```python
from build123d import *

# Parameters (mm, degrees)
SKETCH1_R           = 11
SKETCH1_R_2         = 9.652
BOSS_EXTRUDE1_DEPTH = 15
BOSS_EXTRUDE2_START = 1.5
SKETCH2_R           = 11
BOSS_EXTRUDE2_DEPTH = 1.5
SKETCH4_W           = 5
SKETCH4_H           = 12
BOSS_EXTRUDE4_DEPTH = 35
SKETCH5_R           = 4
CUT_EXTRUDE1_DEPTH  = 5
CUT_EXTRUDE2_DEPTH  = 41.441315508
FILLET1_R           = 4


with BuildPart() as part:
    # Sketch1 → Boss-Extrude1 (new body)
    with BuildSketch(Plane(origin=(0, 0, 0), x_dir=(1, 0, 0), z_dir=(0, 1, 0))):
        with Locations(Location((0, 0, 0), (0, 0, 270))):
            Circle(SKETCH1_R)
        with Locations(Location((0, 0, 0), (0, 0, 270))):
            Circle(SKETCH1_R_2, mode=Mode.SUBTRACT)
    extrude(amount=BOSS_EXTRUDE1_DEPTH)

    # Sketch2 → Boss-Extrude2 (add)
    with BuildSketch(Plane.XZ.offset(BOSS_EXTRUDE2_START)):
        with Locations(Location((0, 0, 0), (0, 0, 270))):
            Circle(SKETCH2_R)
    extrude(amount=-BOSS_EXTRUDE2_DEPTH)

    # Sketch4 → Boss-Extrude4 (add)
    with BuildSketch(Plane.XZ.offset(1.5)):
        Rectangle(SKETCH4_W, SKETCH4_H)
    extrude(amount=BOSS_EXTRUDE4_DEPTH)

    # Sketch5 → Cut-Extrude1 (cut)
    with BuildSketch(Plane.ZY.offset(2.5)):
        with Locations((0, -30.5)):
            Circle(SKETCH5_R)
    extrude(amount=-CUT_EXTRUDE1_DEPTH, mode=Mode.SUBTRACT)

    # Sketch6 → Cut-Extrude2 (cut, through all)
    with BuildSketch(Plane.ZY.offset(2.5)):
        with BuildLine():
            Line((-6, -30.5), (-6, -36.5))
            ThreePointArc((-6, -36.5), (0, -38.985281374), (6, -36.5))
            Line((6, -36.5), (6, -30.5))
            ThreePointArc((6, -30.5), (0, -36.5), (-6, -30.5))
        make_face()
    extrude(amount=-CUT_EXTRUDE2_DEPTH, mode=Mode.SUBTRACT)

    # Fillet1
    # the kernel refuses this fillet: 4 mm, written as the material it adds along each edge
    with BuildSketch(Plane(origin=(2.5, -1.5, -6), x_dir=(1, 0, 0), z_dir=(0, 0, 1)), Plane(origin=(-2.5, -1.5, 6), x_dir=(-1, 0, 0), z_dir=(0, 0, -1))) as fillet1_piece_1:
        with BuildLine():
            CenterArc((FILLET1_R, -FILLET1_R), FILLET1_R, 90, 90)
            Line((0, -FILLET1_R), (0, 0))
            Line((0, 0), (FILLET1_R, 0))
        make_face()
    extrude(amount=12)
    with BuildSketch(Plane(origin=(2.5, -1.5, 6), x_dir=(0, 0, 1), z_dir=(-1, 0, 0)), Plane(origin=(-2.5, -1.5, -6), x_dir=(0, 0, -1), z_dir=(1, 0, 0))) as fillet1_piece_2:
        with BuildLine():
            CenterArc((FILLET1_R, -FILLET1_R), FILLET1_R, 90, 90)
            Line((0, -FILLET1_R), (0, 0))
            Line((0, 0), (FILLET1_R, 0))
        make_face()
    extrude(amount=5)
    with BuildSketch(Plane(origin=(-2.5, -1.5, -6), x_dir=(0, 0, -1), z_dir=(1, 0, 0))) as fillet1_piece_3a_section:
        with BuildLine():
            CenterArc((FILLET1_R, -FILLET1_R), FILLET1_R, 90, 90)
            Line((0, -FILLET1_R), (0, 0))
            Line((0, 0), (FILLET1_R, 0))
        make_face()
    fillet1_piece_3a = extrude(amount=15, mode=Mode.PRIVATE)
    fillet1_piece_3a = fillet1_piece_3a & Plane(origin=(0, -2.470762695, 0), x_dir=(0, 0, -1), z_dir=(0, -1, 0)) * Cylinder(11, 46, mode=Mode.PRIVATE)
    fillet1_piece_3a = split(fillet1_piece_3a, bisect_by=Plane(origin=(2.5, -2.470762695, -6.788618782), z_dir=(1, 0, 0)), keep=Keep.TOP, mode=Mode.PRIVATE)
    with BuildSketch(Plane(origin=(2.5, -1.5, -16), x_dir=(1, 0, 0), z_dir=(0, 0, 1))) as fillet1_piece_3b_section:
        with BuildLine():
            CenterArc((FILLET1_R, -FILLET1_R), FILLET1_R, 90, 90)
            Line((0, -FILLET1_R), (0, 0))
            Line((0, 0), (FILLET1_R, 0))
        make_face()
    fillet1_piece_3b = extrude(amount=22, mode=Mode.PRIVATE)
    fillet1_piece_3b = fillet1_piece_3b & Plane(origin=(0, -2.441237168, 0), x_dir=(0, 0, -1), z_dir=(0, -1, 0)) * Cylinder(11, 60, mode=Mode.PRIVATE)
    fillet1_piece_3b = split(fillet1_piece_3b, bisect_by=Plane(origin=(3.34113706, -2.441237168, -6), z_dir=(0, 0, -1)), keep=Keep.TOP, mode=Mode.PRIVATE)
    fillet1_piece_3 = fillet1_piece_3a & fillet1_piece_3b
    add(fillet1_piece_3)
    with BuildSketch(Plane(origin=(2.5, -1.5, -6), x_dir=(1, 0, 0), z_dir=(0, 0, 1))) as fillet1_piece_4a_section:
        with BuildLine():
            CenterArc((FILLET1_R, -FILLET1_R), FILLET1_R, 90, 90)
            Line((0, -FILLET1_R), (0, 0))
            Line((0, 0), (FILLET1_R, 0))
        make_face()
    fillet1_piece_4a = extrude(amount=22, mode=Mode.PRIVATE)
    fillet1_piece_4a = fillet1_piece_4a & Plane(origin=(0, -2.441236356, 0), x_dir=(0, 0, -1), z_dir=(0, -1, 0)) * Cylinder(11, 60, mode=Mode.PRIVATE)
    fillet1_piece_4a = split(fillet1_piece_4a, bisect_by=Plane(origin=(3.341136574, -2.441236356, 6), z_dir=(0, 0, 1)), keep=Keep.TOP, mode=Mode.PRIVATE)
    with BuildSketch(Plane(origin=(12.5, -1.5, 6), x_dir=(0, 0, 1), z_dir=(-1, 0, 0))) as fillet1_piece_4b_section:
        with BuildLine():
            CenterArc((FILLET1_R, -FILLET1_R), FILLET1_R, 90, 90)
            Line((0, -FILLET1_R), (0, 0))
            Line((0, 0), (FILLET1_R, 0))
        make_face()
    fillet1_piece_4b = extrude(amount=15, mode=Mode.PRIVATE)
    fillet1_piece_4b = fillet1_piece_4b & Plane(origin=(0, -2.470761842, 0), x_dir=(0, 0, -1), z_dir=(0, -1, 0)) * Cylinder(11, 46, mode=Mode.PRIVATE)
    fillet1_piece_4b = split(fillet1_piece_4b, bisect_by=Plane(origin=(2.5, -2.470761842, 6.78861866), z_dir=(1, 0, 0)), keep=Keep.TOP, mode=Mode.PRIVATE)
    fillet1_piece_4 = fillet1_piece_4a & fillet1_piece_4b
    add(fillet1_piece_4)
    with BuildSketch(Plane(origin=(2.5, -1.5, 6), x_dir=(0, 0, 1), z_dir=(-1, 0, 0))) as fillet1_piece_5a_section:
        with BuildLine():
            CenterArc((FILLET1_R, -FILLET1_R), FILLET1_R, 90, 90)
            Line((0, -FILLET1_R), (0, 0))
            Line((0, 0), (FILLET1_R, 0))
        make_face()
    fillet1_piece_5a = extrude(amount=15, mode=Mode.PRIVATE)
    fillet1_piece_5a = fillet1_piece_5a & Plane(origin=(0, -2.470762695, 0), x_dir=(0, 0, -1), z_dir=(0, -1, 0)) * Cylinder(11, 46, mode=Mode.PRIVATE)
    fillet1_piece_5a = split(fillet1_piece_5a, bisect_by=Plane(origin=(-2.5, -2.470762695, 6.788618782), z_dir=(-1, 0, 0)), keep=Keep.TOP, mode=Mode.PRIVATE)
    with BuildSketch(Plane(origin=(-2.5, -1.5, 16), x_dir=(-1, 0, 0), z_dir=(0, 0, -1))) as fillet1_piece_5b_section:
        with BuildLine():
            CenterArc((FILLET1_R, -FILLET1_R), FILLET1_R, 90, 90)
            Line((0, -FILLET1_R), (0, 0))
            Line((0, 0), (FILLET1_R, 0))
        make_face()
    fillet1_piece_5b = extrude(amount=22, mode=Mode.PRIVATE)
    fillet1_piece_5b = fillet1_piece_5b & Plane(origin=(0, -2.441237168, 0), x_dir=(0, 0, -1), z_dir=(0, -1, 0)) * Cylinder(11, 60, mode=Mode.PRIVATE)
    fillet1_piece_5b = split(fillet1_piece_5b, bisect_by=Plane(origin=(-3.34113706, -2.441237168, 6), z_dir=(0, 0, 1)), keep=Keep.TOP, mode=Mode.PRIVATE)
    fillet1_piece_5 = fillet1_piece_5a & fillet1_piece_5b
    add(fillet1_piece_5)
    with BuildSketch(Plane(origin=(-12.5, -1.5, -6), x_dir=(0, 0, -1), z_dir=(1, 0, 0))) as fillet1_piece_6a_section:
        with BuildLine():
            CenterArc((FILLET1_R, -FILLET1_R), FILLET1_R, 90, 90)
            Line((0, -FILLET1_R), (0, 0))
            Line((0, 0), (FILLET1_R, 0))
        make_face()
    fillet1_piece_6a = extrude(amount=15, mode=Mode.PRIVATE)
    fillet1_piece_6a = fillet1_piece_6a & Plane(origin=(0, -2.470761842, 0), x_dir=(0, 0, -1), z_dir=(0, -1, 0)) * Cylinder(11, 46, mode=Mode.PRIVATE)
    fillet1_piece_6a = split(fillet1_piece_6a, bisect_by=Plane(origin=(-2.5, -2.470761842, -6.788618661), z_dir=(-1, 0, 0)), keep=Keep.TOP, mode=Mode.PRIVATE)
    with BuildSketch(Plane(origin=(-2.5, -1.5, 6), x_dir=(-1, 0, 0), z_dir=(0, 0, -1))) as fillet1_piece_6b_section:
        with BuildLine():
            CenterArc((FILLET1_R, -FILLET1_R), FILLET1_R, 90, 90)
            Line((0, -FILLET1_R), (0, 0))
            Line((0, 0), (FILLET1_R, 0))
        make_face()
    fillet1_piece_6b = extrude(amount=22, mode=Mode.PRIVATE)
    fillet1_piece_6b = fillet1_piece_6b & Plane(origin=(0, -2.441236356, 0), x_dir=(0, 0, -1), z_dir=(0, -1, 0)) * Cylinder(11, 60, mode=Mode.PRIVATE)
    fillet1_piece_6b = split(fillet1_piece_6b, bisect_by=Plane(origin=(-3.341136574, -2.441236356, -6), z_dir=(0, 0, -1)), keep=Keep.TOP, mode=Mode.PRIVATE)
    fillet1_piece_6 = fillet1_piece_6a & fillet1_piece_6b
    add(fillet1_piece_6)


solid = part.part
```
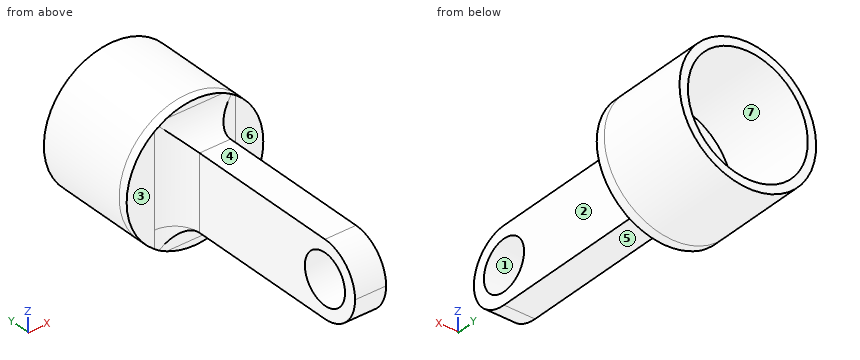
Geometry check sheet. Reference: the model listing, model coordinates, mm. Face numbers are marked on the shaded views. A direction names the side the tool comes from. Round coordinates to 2 decimals unless told otherwise and drop trailing zeros. Loops run counter-clockwise (first coordinate to the right, second up) from the corner with the lowest first, then second, coordinate; pieces in that order, holes last. Notation, with made-up numbers: (2, 3) - (28, 3) arc R24 ccw to (28, 21) - close; hole circle Ø6 at (23.25, 29.5). An arc over 180 degrees is marked (long way). Write item = value, one per line. Start each with the question number.
1. Mould release check, pull along Z, two halves, no side actions. Record for the marked faces 5, 6 and 7: released by +Z, released by -Z, zero draft, split by the parting line, or undercut.
2. Section check C-C on z = 8. Enter the section's corners in (x, y).
3. Section check B-B on y = -27.5. Enter the section's corners in (x, z), then the cut area to 3 significant figures.
4. Section check A-A on x = 0. Enter the section's corners in (y, z).
5. Section check D-D on y = -11.5. Enter the section's corners in (x, z).
6. Depth check by flat-ended pin: pin 1 (1.1 mm diameter, centred on x = -1, z = 10.5, fed in from -Y); pin 2 (1.5 mm diameter, centred on x = 3, y = -28.5, fed in from +Z); pin 3 (1.5 mm diameter, centred on x = 5.5, y = -4, fed in from -Z); pin 4 (1.5 mm diameter, centred on x = -1, y = -19.5, fed in from -Z). Enter the tip coordinate at first touch or a pass-through.
7. Thickness scan on line 1 (X direction, y = 5, z = 0); line 2 (Y direction, x = 0.1, z = 0); line 3 (Z direction, x = 8, y = 5). Record the ranges inside material, lowest first.
8. Set-up check for the marked faces 1, 2, 3 and 4: record each of +Z, -Z, +X, -X, +Y, -Y from which the full face is reachable in a straight line by a thin tool's end or side.
Working result:
q1.face_5 = released by -Z
q1.face_6 = zero draft
q1.face_7 = undercut
q2.outline = (-7.55, -1.5) - (-6.5, -1.5) arc R4 cw to (-4.5, -2.04) - (4.5, -2.04) arc R4 cw to (6.5, -1.5) - (7.55, -1.5) - (7.55, 15) - (5.4, 15) - (5.4, 0) - (-5.4, 0) - (-5.4, 15) - (-7.55, 15) - close
q3.outline = (-2.5, -6) - (2.5, -6) - (2.5, -2.65) - (-2.5, -2.65) - close; (-2.5, 2.65) - (2.5, 2.65) - (2.5, 6) - (-2.5, 6) - close
q3.area = 33.5 mm^2
q4.outline = (-30.5, -6) - (-5.5, -6) arc R4 cw to (-1.5, -10) - (-1.5, -11) - (15, -11) - (15, -9.65) - (0, -9.65) - (0, 9.65) - (15, 9.65) - (15, 11) - (-1.5, 11) - (-1.5, 10) arc R4 cw to (-5.5, 6) - (-30.5, 6) arc R6 ccw to start; hole circle Ø8 at (-30.5, 0)
q5.outline = (-2.5, -6) - (2.5, -6) - (2.5, 6) - (-2.5, 6) - close
q6.pin_1 = -1.5
q6.pin_2 = 6
q6.pin_3 = through
q6.pin_4 = -6
q7.line_1 = -11 to -9.65, 9.65 to 11
q7.line_2 = -36.5 to -34.5, -26.5 to 0
q7.line_3 = -7.55 to -5.4, 5.4 to 7.55
q8.face_1 = +X, -X
q8.face_2 = +Z, -Z, +X, -Y
q8.face_3 = +Z, -Z, -X, -Y
q8.face_4 = +Z, +X, -X, -Y
